Model file for the job. Use its own axes, mm. Round coordinates to 2 decimals unless told otherwise and drop trailing zeros. Loops run counter-clockwise (first coordinate to the right, second up) from the corner with the lowest first, then second, coordinate; pieces in that order, holes last. Notation, with made-up numbers: M 64,53.25 L 72,53.25 A13 ccw 72,58.25 Z; hole C 21.5,22.5 d4. An arc over 180 degrees is marked long. Use a Markdown table: item, result. Add a question column.
Q1. Cut at B-B (y = 2.45). Give the cut face in (x, z), plus the area to 3 significant figures.
Q2. Cut at A-A (z = -7.25). Give the cut face in (x, y), plus the area to 3 significant figures.
Q3. Cut at C-C (x = 59.5). Give the cut face in (y, z).
Q4. Probe line 1 (Z direction, x = 74.5, y = 2.35); line 2 (X direction, y = 1.1, z = -4); line 3 (X direction, y = 0.9, z = -2). List the from-to ranges inside material, lowest first. Write a range as from..to.
Q5. Mould opens along X. For faces 1 (the face through (67, 0, -6)), 2 (the face through (136.8, 1, -6)), 3 (the face through (69, 1, -6)) say: +X half, -X half, draft (parallel to the pull), parting line (faces both ways), or undercut.
Q6. Pin check, flat tips, straight feed: pin 1 (3 mm diameter, centred on x = 91.5, z = -5.5, fed in from +Y); pin 2 (0.6 mm diameter, centred on x = 0.5, y = 2.5, fed in from +Z); pin 3 (0.6 mm diameter, centred on y = 2, z = -11.5, fed in from -X). Stop position of each tip, or through.
from build123d import *

# Parameters (mm, degrees)
ESQUISSE1_W             = 136.8
ESQUISSE1_H             = 11.8
BOSS_EXTRU_1_DEPTH      = 1
ESQUISSE4_W             = 136.8
ESQUISSE4_H             = 11.8
ESQUISSE4_W_2           = 135.2
ESQUISSE4_H_2           = 10.2
BOSS_EXTRU_3_DEPTH      = 2
ESQUISSE5_W             = 4.4
ESQUISSE5_H             = 0.8
ENL_V_MAT_EXTRU_3_DEPTH = 2
ESQUISSE6_W             = 3
ESQUISSE6_H             = 8.8
ENL_V_MAT_EXTRU_4_DEPTH = 4
CONG_1_R                = 1


with BuildPart() as part:
    # Esquisse1 → Boss.-Extru.1 (new body)
    with BuildSketch(Plane(origin=(0, 0, 0), x_dir=(1, 0, 0), z_dir=(0, 1, 0))):
        with Locations((68.4, 5.9)):
            Rectangle(ESQUISSE1_W, ESQUISSE1_H)
    extrude(amount=BOSS_EXTRU_1_DEPTH)

    # Esquisse4 → Boss.-Extru.3 (add)
    with BuildSketch(Plane(origin=(0, 1, 0), x_dir=(1, 0, 0), z_dir=(0, 1, 0))):
        with Locations((68.4, 5.9)):
            Rectangle(ESQUISSE4_W, ESQUISSE4_H)
        with Locations((68.4, 5.9)):
            Rectangle(ESQUISSE4_W_2, ESQUISSE4_H_2, mode=Mode.SUBTRACT)
    extrude(amount=BOSS_EXTRU_3_DEPTH)

    # Esquisse5 → Enlèv. mat.-Extru.3 (cut)
    with BuildSketch(Plane(origin=(0, 3, 0), x_dir=(1, 0, 0), z_dir=(0, 1, 0))):
        Polygon((136.8, 11.8), (136.8, 8.4), (136, 8.4), (136, 11), (133.4, 11), (133.4, 11.8), align=None)
        Polygon((3.4, 11.8), (0, 11.8), (0, 8.4), (0.8, 8.4), (0.8, 11), (3.4, 11), align=None)
        with Locations((68.4, 11.4)):
            Rectangle(ESQUISSE5_W, ESQUISSE5_H)
        Polygon((0, 0), (0, 3.4), (0.8, 3.4), (0.8, 0.8), (3.4, 0.8), (3.4, 0), align=None)
        with Locations((68.4, 0.4)):
            Rectangle(ESQUISSE5_W, ESQUISSE5_H)
        Polygon((133.4, 0), (136.8, 0), (136.8, 3.4), (136, 3.4), (136, 0.8), (133.4, 0.8), align=None)
    extrude(amount=-ENL_V_MAT_EXTRU_3_DEPTH, mode=Mode.SUBTRACT)

    # Esquisse6 → Enlèv. mat.-Extru.4 (cut, through all)
    with BuildSketch(Plane.XZ):
        with Locations((3, -5.9)):
            Rectangle(ESQUISSE6_W, ESQUISSE6_H)
    extrude(amount=-ENL_V_MAT_EXTRU_4_DEPTH, mode=Mode.SUBTRACT)

    # Congé1
    cong_1_edges = [part.edges().sort_by_distance(p)[0] for p in [
        (0, 0.5, -11.8),
        (136.8, 0.5, -11.8),
        (136.8, 0.5, 0),
        (0, 0.5, 0),
    ]]
    fillet(cong_1_edges, radius=CONG_1_R)


solid = part.part
Checked values:
| question | item | result |
|---|---|---|
| 1 | outline | M 0,-8.4 L 0.8,-8.4 L 0.8,-3.4 L 0,-3.4 Z; M 3.4,-11.8 L 66.2,-11.8 L 66.2,-11 L 3.4,-11 Z; M 3.4,-0.8 L 66.2,-0.8 L 66.2,0 L 3.4,0 Z; M 70.6,-11.8 L 133.4,-11.8 L 133.4,-11 L 70.6,-11 Z; M 70.6,-0.8 L 133.4,-0.8 L 133.4,0 L 70.6,0 Z; M 136,-8.4 L 136.8,-8.4 L 136.8,-3.4 L 136,-3.4 Z |
| 1 | area | 209 mm^2 |
| 2 | outline | M 0,0 L 1.5,0 L 1.5,1 L 0.8,1 L 0.8,3 L 0,3 Z; M 4.5,0 L 136.8,0 L 136.8,3 L 136,3 L 136,1 L 4.5,1 Z |
| 2 | area | 137 mm^2 |
| 3 | outline | M 0,-11.8 L 3,-11.8 L 3,-11 L 1,-11 L 1,-0.8 L 3,-0.8 L 3,0 L 0,0 Z |
| 4 | line 1 | z = -11.8..-11, -0.8..0 |
| 4 | line 2 | x = 0..0.8, 136..136.8 |
| 4 | line 3 | x = 0..1.5, 4.5..136.8 |
| 5 | face 1 | draft |
| 5 | face 2 | +X half |
| 5 | face 3 | undercut |
| 6 | pin 1 | stops at y = 1 |
| 6 | pin 2 | stops at z = -3.4 |
| 6 | pin 3 | stops at x = 3.4 |
